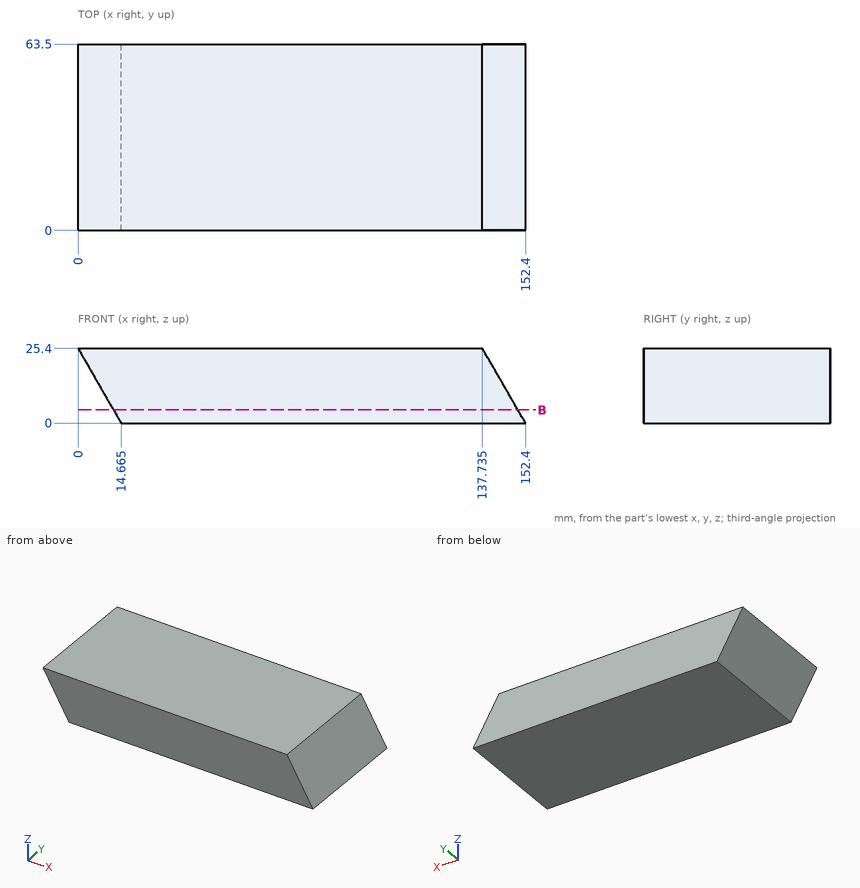
Drawing for the job (mm, zero at the part's lowest x, y, z). Round coordinates to 2 decimals unless told otherwise and drop trailing zeros. Write each loop counter-clockwise with the first axis right and the second up, starting at its lowest first coordinate (ties: lowest second). Pieces come first, ordered by that corner, then holes.
Item 1: Drill centre lines: L1, parallel to X at y = 36, z = 9 (1 decimal); L2, parallel to X at y = 31.5, z = 6 (1 decimal); L3, parallel to Z at x = 138.5, y = 31 (1 decimal). Where is each one in solid material? Low to high.
Filled in:
L1: x = 9.5 to 147.2
L2: x = 11.2 to 148.9
L3: z = 0 to 24.1
Item 2: Drop a flat-ended pin along its axis: pin 1 Ø4 at (y, z) = (48.5, 17.5) entering from -X. Give the stop position or say it passes through.
Filled in:
pin 1: stops at x = 3.41
Item 3: Band-saw the part on B-B on z = 4.5. Write the cut outline in (x, y), then the cut area to 3 significant figures.
Filled in:
outline: (12.07, 0) - (149.8, 0) - (149.8, 63.5) - (12.07, 63.5) - close
area: 8,750 mm2
